Verification items for this drawing (mm, ordinates from the low corner). Give positions to 0.01 mm unless a question says otherwise; leave off trailing zeros. Loops run counter-clockwise (first coordinate to the right, second up) from the corner with the lowest first, then second, coordinate; pieces in that order, holes last. Notation, with made-up numbers: (20.25, -25.75) -> (61.25, -25.75) arc R12 cw to (61.25, -8.75) -> close; hole circle Ø11 at (5.25, 34). An arc over 180 degrees is marked (long way). Answer in a Markdown table with one row per item. Add a question column.
Q1. Section check D-D on z = 163.5. Enter the section's corners in (x, y), and give its area (3 significant figures).
Q2. Section check A-A on z = 85. Enter the section's corners in (x, y) (3 decimals).
Q3. Gauge pin test, flat ends, axial feed: P1, Ø3.5, axis at x = 29.49, z = 29.49, coming from the -Y side; P2, Ø1, axis at y = 0, z = 105.5, coming from the +X side. Record the tip position at first contact, or that the pin passes through.
Q4. Material ranges on probe 1 along X at (y, z) = (0.8, 85) (3 decimals); probe 2 along X at (y, z) = (0.4, 142) (1 decimal); probe 3 along Z at (x, y) = (83.5, 1.1), recorded low to high.
Q5. Section check B-B on x = 85. Enter the section's corners in (y, z) (3 decimals).
Q6. Section check C-C on y = 0.95. Give the number of separate pieces and of enclosed holes in the cut face, and give its area (3 significant figures).
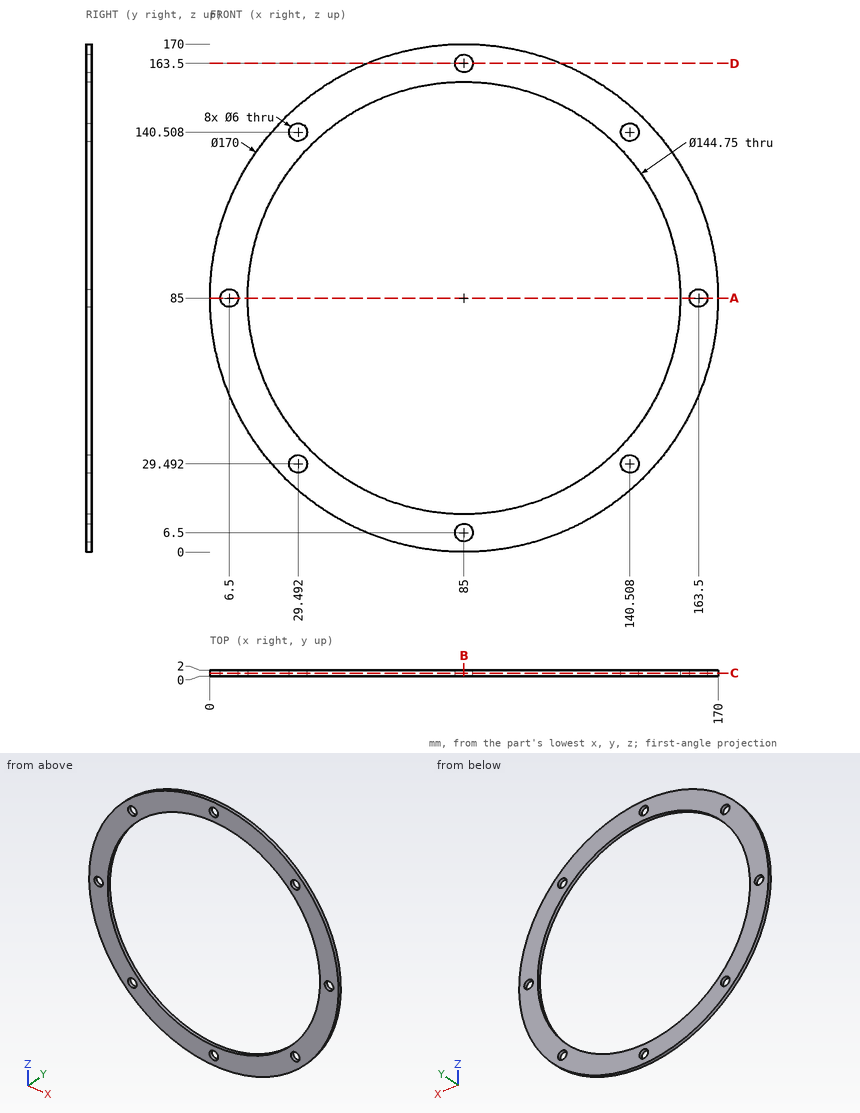
Taken from the geometry:
| question | item | result |
|---|---|---|
| 1 | outline | (52.4, 0) -> (82, 0) -> (82, 2) -> (52.4, 2) -> close; (88, 0) -> (117.6, 0) -> (117.6, 2) -> (88, 2) -> close |
| 1 | area | 118 mm² |
| 2 | outline | (0, 0) -> (3.5, 0) -> (3.5, 2) -> (0, 2) -> close; (9.5, 0) -> (12.625, 0) -> (12.625, 2) -> (9.5, 2) -> close; (157.375, 0) -> (160.5, 0) -> (160.5, 2) -> (157.375, 2) -> close; (166.5, 0) -> (170, 0) -> (170, 2) -> (166.5, 2) -> close |
| 3 | P1 | passes through |
| 3 | P2 | stops at x = 167.61 |
| 4 | probe 1 | x = 0 to 3.5, 9.5 to 12.625, 157.375 to 160.5, 166.5 to 170 |
| 4 | probe 2 | x = 21.9 to 26.9, 32.1 to 40.4, 129.6 to 137.9, 143.1 to 148.1 |
| 4 | probe 3 | z = 0.01 to 3.9, 9.1 to 12.64, 157.36 to 160.9, 166.1 to 169.99 |
| 5 | outline | (0, 0) -> (2, 0) -> (2, 3.5) -> (0, 3.5) -> close; (0, 9.5) -> (2, 9.5) -> (2, 12.625) -> (0, 12.625) -> close; (0, 157.375) -> (2, 157.375) -> (2, 160.5) -> (0, 160.5) -> close; (0, 166.5) -> (2, 166.5) -> (2, 170) -> (0, 170) -> close |
| 6 | separate pieces | 1 |
| 6 | enclosed holes | 9 |
| 6 | area | 6,020 mm² |
